Could you check a few things on this model? Use its own coordinates, in mm. Face numbers are marked on the shaded views. A direction names the side the tool comes from. Give positions to 0.01 mm unless a question says otherwise; leave off trailing zeros. Loops run counter-clockwise (first coordinate to the right, second up) from the corner with the lowest first, then second, coordinate; pieces in that order, holes last. Notation, with made-up numbers: M 66,71 L 80,71 A10 ccw 80,82 Z; hole C -11.75,40 d10. An arc over 180 degrees is marked long. Use CSV: the item, a comma, the result in double quotes.
```python
from build123d import *

# Parameters (mm, degrees)
SKETCH2_R               = 15
BOSS_EXTRUDE1_DEPTH     = 15
BOSS_EXTRUDE1_2_DEPTH   = 15
BOSS_EXTRUDE2_DEPTH     = 140
CUT_EXTRUDE2_DEPTH      = 261.480325553
CUT_EXTRUDE2_DEPTH_BACK = 261.480325553
SKETCH4_R               = 15


with BuildPart() as part:
    # Sketch2 → Boss-Extrude1 (new body)
    with BuildSketch(Plane(origin=(0, 0, 0), x_dir=(1, 0, 0), z_dir=(0, 1, 0))):
        with BuildLine():
            Line((-140, -90), (-140, 90))
            ThreePointArc((-140, 90), (-110, 120), (-80, 90))
            Line((-80, 90), (-80, -90))
            ThreePointArc((-80, -90), (-110, -120), (-140, -90))
        make_face()
        with Locations(Location((-110, 90, 0), (0, 0, 270))):
            Circle(SKETCH2_R, mode=Mode.SUBTRACT)
        with Locations(Location((-110, -90, 0), (0, 0, 270))):
            Circle(SKETCH2_R, mode=Mode.SUBTRACT)
    extrude(amount=BOSS_EXTRUDE1_DEPTH)



with BuildPart() as body_2:
    # Sketch2 → Boss-Extrude1 2 (new body)
    with BuildSketch(Plane(origin=(0, 0, 0), x_dir=(1, 0, 0), z_dir=(0, 1, 0))):
        with BuildLine():
            Line((140, -90), (140, 90))
            ThreePointArc((140, 90), (110, 120), (80, 90))
            Line((80, 90), (80, -90))
            ThreePointArc((80, -90), (110, -120), (140, -90))
        make_face()
        with Locations(Location((110, -90, 0), (0, 0, 90))):
            Circle(SKETCH2_R, mode=Mode.SUBTRACT)
        with Locations(Location((110, 90, 0), (0, 0, 90))):
            Circle(SKETCH2_R, mode=Mode.SUBTRACT)
    extrude(amount=BOSS_EXTRUDE1_2_DEPTH)


with BuildPart() as part_1:
    add(part.part)

    add(body_2.part)  # Boss-Extrude2 merges body 2
    # Sketch3 → Boss-Extrude2 (add, symmetric)
    with BuildSketch(Plane(origin=(0, 0, 0), x_dir=(0, 0, -1), z_dir=(1, 0, 0))):
        with BuildLine():
            Line((-10, 165), (-10, 93.729833462))
            ThreePointArc((-10, 93.729833462), (0, 15), (10, 93.729833462))
            Line((10, 93.729833462), (10, 165))
            Line((10, 165), (25, 165))
            Line((25, 165), (25, 103.989794856))
            ThreePointArc((25, 103.989794856), (0, 0), (-25, 103.989794856))
            Line((-25, 103.989794856), (-25, 165))
            Line((-25, 165), (-10, 165))
        make_face()
    extrude(amount=BOSS_EXTRUDE2_DEPTH, both=True)

    # Sketch4 → Cut-Extrude2 (cut, two sides: drawn at the far end of the back side and taken through both)
    with BuildSketch(Plane.XY.offset(25).offset(-CUT_EXTRUDE2_DEPTH_BACK)):
        with BuildLine():
            Line((-140, 165), (-140, 103.989794856))
            Line((-140, 103.989794856), (-100, 103.989794856))
            Line((-100, 103.989794856), (-100, 135))
            ThreePointArc((-100, 135), (-91.213203436, 156.213203436), (-70, 165))
            Line((-70, 165), (-140, 165))
        make_face()
        with Locations(Location((-70, 135, 0), (0, 0, 90))):
            Circle(SKETCH4_R)
        with BuildLine():
            Line((-40, 135), (-40, 103.989794856))
            Line((-40, 103.989794856), (0, 103.989794856))
            Line((0, 103.989794856), (0, 165))
            Line((0, 165), (-70, 165))
            ThreePointArc((-70, 165), (-48.786796564, 156.213203436), (-40, 135))
        make_face()
        with BuildLine():
            Line((0, 165), (0, 103.989794856))
            Line((0, 103.989794856), (40, 103.989794856))
            Line((40, 103.989794856), (40, 135))
            ThreePointArc((40, 135), (48.786796564, 156.213203436), (70, 165))
            Line((70, 165), (0, 165))
        make_face()
        with Locations(Location((70, 135, 0), (0, 0, 90))):
            Circle(SKETCH4_R)
        with BuildLine():
            Line((140, 165), (70, 165))
            ThreePointArc((70, 165), (91.213203436, 156.213203436), (100, 135))
            Line((100, 135), (100, 103.989794856))
            Line((100, 103.989794856), (140, 103.989794856))
            Line((140, 103.989794856), (140, 165))
        make_face()
    extrude(amount=CUT_EXTRUDE2_DEPTH + CUT_EXTRUDE2_DEPTH_BACK, mode=Mode.SUBTRACT)


solid = part_1.part
```
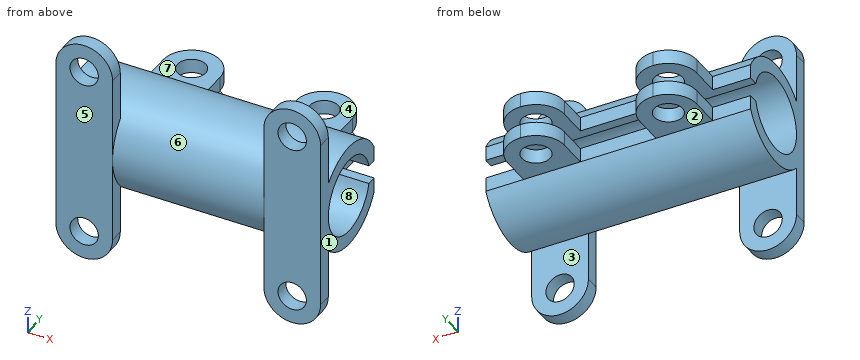
1. I'm going to push flat-ended pins straight in: pin 1 Ø10 at (x, y) = (-39.5, 39.5) entering from +Z; pin 2 Ø4.5 at (x, z) = (-123.5, -21) entering from +Y; pin 3 Ø8 at (x, y) = (43, 98) entering from +Z. Where does each tip first touch, or does it pass through?
Outcome:
pin 1,"z = 53.99"
pin 2,"y = 103.99"
pin 3,"z = 38.78"
2. Please list where these lines run through material, in increasing order: line 1 (X direction, y = 135, z = -15); line 2 (Z direction, x = 109.5, y = 9); line 3 (Z direction, x = 7, y = 95).
Outcome:
line 1,"-100 to -85, -55 to -40, 40 to 55, 85 to 100"
line 2,"-120 to -104.99, -75.01 to 75.01, 104.99 to 120"
line 3,"-37.75 to -10, 10 to 37.75"
3. I want a section at C-C, the plane z = 43.5. List the corners of the cut face in (x, y) for me, then the cut area to 3 significant figures.
Outcome:
outline,"M -140,0 L -80,0 L -80,15 L -140,15 Z; M -140,21.34 L 140,21.34 L 140,88.66 L -140,88.66 Z; M 80,0 L 140,0 L 140,15 L 80,15 Z"
area,"20,600 mm2"
4. I want a section at D-D, the plane x = 4. List the corners of the cut face in (y, z) for me, then the cut area to 3 significant figures.
Outcome:
outline,"M 93.73,-10 A40 cw long 93.73,10 L 103.99,10 L 103.99,25 A55 ccw long 103.99,-25 L 103.99,-10 Z"
area,"4,090 mm2"
5. I want a section at B-B, the plane y = 55. List the corners of the cut face in (x, z) for me, then the cut area to 3 significant figures.
Outcome:
outline,"M -140,-55 L 140,-55 L 140,-40 L -140,-40 Z; M -140,40 L 140,40 L 140,55 L -140,55 Z"
area,"8,400 mm2"
6. I want a section at A-A, the plane x = -110. List the corners of the cut face in (y, z) for me, then the cut area to 3 significant figures.
Outcome:
outline,"M 0,-120 L 15,-120 L 15,-105 L 0,-105 Z; M 0,-75 L 15,-75 L 15,-37.75 A55 ccw 103.99,-25 L 103.99,-10 L 93.73,-10 A40 cw long 93.73,10 L 103.99,10 L 103.99,25 A55 ccw 15,37.75 L 15,75 L 0,75 Z; M 0,105 L 15,105 L 15,120 L 0,120 Z"
area,"6,010 mm2"
7. Which directions (+Z, -Z, +X, -X, +Y, -Y) give clear straight access to the entire face, cutting with the end or side of a thin tool? Please do the marked faces 1, 2, 3 and 4.
Outcome:
face 1,"+Z, -Z, +X, +Y, -Y"
face 2,"-Z, +X, -X, +Y"
face 3,"-Z, +X, -X"
face 4,"+Z, +X, -X, +Y"
8. If we mould it in two halves opening along Z, with no side actions, what happens to the marked faces 5, 6, 7 and 8? For each: +Z half, -Z half, draft (parallel to the pull), parting line (faces both ways), or undercut.
Outcome:
face 5,"draft"
face 6,"parting line"
face 7,"+Z half"
face 8,"undercut"
